from build123d import *

# Parameters (mm, degrees)
F0_W     = 30
F0_H     = 30
F1_DEPTH = 1.6
F3_DEPTH = 15
F4_DEPTH = 25


with BuildPart() as f1:
    # F0 (on Top) → F1 (new body)
    with BuildSketch(Plane.XY):
        with Locations((15, -15)):
            Rectangle(F0_W, F0_H)
    extrude(amount=F1_DEPTH)

    # F2 (on face) → F3 (join)
    with BuildSketch(Plane.XY.offset(1.6)):
        with BuildLine():
            Line((5.8029437252, -5.8029437252), (4.6715728753, -4.6715728753))
            ThreePointArc((4.6715728753, -4.6715728753), (3.5, -7.5), (4.6715728753, -10.3284271247))
            Line((4.6715728753, -10.3284271247), (5.8029437252, -9.1970562748))
            ThreePointArc((5.8029437252, -9.1970562748), (5.1, -7.5), (5.8029437252, -5.8029437252))
        make_face()
        with BuildLine():
            ThreePointArc((10.3284271247, -4.6715728753), (7.5, -3.5), (4.6715728753, -4.6715728753))
            Line((4.6715728753, -4.6715728753), (5.8029437252, -5.8029437252))
            ThreePointArc((5.8029437252, -5.8029437252), (7.5, -5.1), (9.1970562748, -5.8029437252))
            Line((9.1970562748, -5.8029437252), (10.3284271247, -4.6715728753))
        make_face()
        with BuildLine():
            ThreePointArc((11.5, -7.5), (11.19551813, -5.9692662705), (10.3284271247, -4.6715728753))
            Line((10.3284271247, -4.6715728753), (9.1970562748, -5.8029437252))
            ThreePointArc((9.1970562748, -5.8029437252), (9.717310878, -6.5815597623), (9.9, -7.5))
            ThreePointArc((9.9, -7.5), (9.717310878, -8.4184402377), (9.1970562748, -9.1970562748))
            Line((9.1970562748, -9.1970562748), (10.3284271247, -10.3284271247))
            ThreePointArc((10.3284271247, -10.3284271247), (11.19551813, -9.0307337295), (11.5, -7.5))
        make_face()
        with BuildLine():
            Line((5.8029437252, -9.1970562748), (4.6715728753, -10.3284271247))
            ThreePointArc((4.6715728753, -10.3284271247), (7.5, -11.5), (10.3284271247, -10.3284271247))
            Line((10.3284271247, -10.3284271247), (9.1970562748, -9.1970562748))
            ThreePointArc((9.1970562748, -9.1970562748), (7.5, -9.9), (5.8029437252, -9.1970562748))
        make_face()
        with BuildLine():
            ThreePointArc((18.9644660941, -18.9644660941), (17.5, -22.5), (18.9644660941, -26.0355339059))
            Line((18.9644660941, -26.0355339059), (20.095836944, -24.904163056))
            ThreePointArc((20.095836944, -24.904163056), (19.1, -22.5), (20.095836944, -20.095836944))
            Line((20.095836944, -20.095836944), (18.9644660941, -18.9644660941))
        make_face()
        with BuildLine():
            Line((24.904163056, -20.095836944), (26.0355339059, -18.9644660941))
            ThreePointArc((26.0355339059, -18.9644660941), (22.5, -17.5), (18.9644660941, -18.9644660941))
            Line((18.9644660941, -18.9644660941), (20.095836944, -20.095836944))
            ThreePointArc((20.095836944, -20.095836944), (22.5, -19.1), (24.904163056, -20.095836944))
        make_face()
        with BuildLine():
            ThreePointArc((27.5, -22.5), (27.1193976626, -20.5865828382), (26.0355339059, -18.9644660941))
            Line((26.0355339059, -18.9644660941), (24.904163056, -20.095836944))
            ThreePointArc((24.904163056, -20.095836944), (25.6411904105, -21.19887633), (25.9, -22.5))
            ThreePointArc((25.9, -22.5), (25.6411904105, -23.80112367), (24.904163056, -24.904163056))
            Line((24.904163056, -24.904163056), (26.0355339059, -26.0355339059))
            ThreePointArc((26.0355339059, -26.0355339059), (27.1193976626, -24.4134171618), (27.5, -22.5))
        make_face()
        with BuildLine():
            Line((20.095836944, -24.904163056), (18.9644660941, -26.0355339059))
            ThreePointArc((18.9644660941, -26.0355339059), (22.5, -27.5), (26.0355339059, -26.0355339059))
            Line((26.0355339059, -26.0355339059), (24.904163056, -24.904163056))
            ThreePointArc((24.904163056, -24.904163056), (22.5, -25.9), (20.095836944, -24.904163056))
        make_face()
    extrude(amount=F3_DEPTH)

    # F2 (on face) → F4 (cut)
    with BuildSketch(Plane.XY.offset(1.6)):
        with BuildLine():
            Line((26.0355339059, -11.0355339059), (22.5, -7.5))
            Line((22.5, -7.5), (18.9644660941, -11.0355339059))
            ThreePointArc((18.9644660941, -11.0355339059), (22.5, -12.5), (26.0355339059, -11.0355339059))
        make_face()
        with BuildLine():
            Line((22.5, -7.5), (18.9644660941, -3.9644660941))
            ThreePointArc((18.9644660941, -3.9644660941), (17.5, -7.5), (18.9644660941, -11.0355339059))
            Line((18.9644660941, -11.0355339059), (22.5, -7.5))
        make_face()
        with BuildLine():
            ThreePointArc((26.0355339059, -3.9644660941), (22.5, -2.5), (18.9644660941, -3.9644660941))
            Line((18.9644660941, -3.9644660941), (22.5, -7.5))
            Line((22.5, -7.5), (26.0355339059, -3.9644660941))
        make_face()
        with BuildLine():
            Line((26.0355339059, -3.9644660941), (22.5, -7.5))
            Line((22.5, -7.5), (26.0355339059, -11.0355339059))
            ThreePointArc((26.0355339059, -11.0355339059), (27.1193976626, -9.4134171618), (27.5, -7.5))
            ThreePointArc((27.5, -7.5), (27.1193976626, -5.5865828382), (26.0355339059, -3.9644660941))
        make_face()
        with BuildLine():
            Line((9.1970562748, -5.8029437252), (7.5, -7.5))
            Line((7.5, -7.5), (9.1970562748, -9.1970562748))
            ThreePointArc((9.1970562748, -9.1970562748), (9.717310878, -8.4184402377), (9.9, -7.5))
            ThreePointArc((9.9, -7.5), (9.717310878, -6.5815597623), (9.1970562748, -5.8029437252))
        make_face()
        with BuildLine():
            ThreePointArc((9.1970562748, -5.8029437252), (7.5, -5.1), (5.8029437252, -5.8029437252))
            Line((5.8029437252, -5.8029437252), (7.5, -7.5))
            Line((7.5, -7.5), (9.1970562748, -5.8029437252))
        make_face()
        with BuildLine():
            Line((7.5, -7.5), (5.8029437252, -5.8029437252))
            ThreePointArc((5.8029437252, -5.8029437252), (5.1, -7.5), (5.8029437252, -9.1970562748))
            Line((5.8029437252, -9.1970562748), (7.5, -7.5))
        make_face()
        with BuildLine():
            Line((9.1970562748, -9.1970562748), (7.5, -7.5))
            Line((7.5, -7.5), (5.8029437252, -9.1970562748))
            ThreePointArc((5.8029437252, -9.1970562748), (7.5, -9.9), (9.1970562748, -9.1970562748))
        make_face()
        with BuildLine():
            ThreePointArc((10.3284271247, -19.6715728753), (7.5, -18.5), (4.6715728753, -19.6715728753))
            Line((4.6715728753, -19.6715728753), (7.5, -22.5))
            Line((7.5, -22.5), (10.3284271247, -19.6715728753))
        make_face()
        with BuildLine():
            Line((10.3284271247, -19.6715728753), (7.5, -22.5))
            Line((7.5, -22.5), (10.3284271247, -25.3284271247))
            ThreePointArc((10.3284271247, -25.3284271247), (11.19551813, -24.0307337295), (11.5, -22.5))
            ThreePointArc((11.5, -22.5), (11.19551813, -20.9692662705), (10.3284271247, -19.6715728753))
        make_face()
        with BuildLine():
            Line((10.3284271247, -25.3284271247), (7.5, -22.5))
            Line((7.5, -22.5), (4.6715728753, -25.3284271247))
            ThreePointArc((4.6715728753, -25.3284271247), (7.5, -26.5), (10.3284271247, -25.3284271247))
        make_face()
        with BuildLine():
            Line((7.5, -22.5), (4.6715728753, -19.6715728753))
            ThreePointArc((4.6715728753, -19.6715728753), (3.5, -22.5), (4.6715728753, -25.3284271247))
            Line((4.6715728753, -25.3284271247), (7.5, -22.5))
        make_face()
        with BuildLine():
            ThreePointArc((20.095836944, -20.095836944), (19.1, -22.5), (20.095836944, -24.904163056))
            Line((20.095836944, -24.904163056), (22.5, -22.5))
            Line((22.5, -22.5), (20.095836944, -20.095836944))
        make_face()
        with BuildLine():
            Line((22.5, -22.5), (24.904163056, -20.095836944))
            ThreePointArc((24.904163056, -20.095836944), (22.5, -19.1), (20.095836944, -20.095836944))
            Line((20.095836944, -20.095836944), (22.5, -22.5))
        make_face()
        with BuildLine():
            ThreePointArc((25.9, -22.5), (25.6411904105, -21.19887633), (24.904163056, -20.095836944))
            Line((24.904163056, -20.095836944), (22.5, -22.5))
            Line((22.5, -22.5), (24.904163056, -24.904163056))
            ThreePointArc((24.904163056, -24.904163056), (25.6411904105, -23.80112367), (25.9, -22.5))
        make_face()
        with BuildLine():
            Line((22.5, -22.5), (20.095836944, -24.904163056))
            ThreePointArc((20.095836944, -24.904163056), (22.5, -25.9), (24.904163056, -24.904163056))
            Line((24.904163056, -24.904163056), (22.5, -22.5))
        make_face()
    extrude(amount=-F4_DEPTH, mode=Mode.SUBTRACT)


solid = f1.part
Geometry: final body of the model. Coordinates: model frame, mm. A direction names the side the tool comes from. Coordinates: 2 decimals unless noted, no trailing zeros. Order: outer loops, then holes, each group sorted by start corner. A loop starts at its lowest first (then second) coordinate and runs counter-clockwise, first axis right, second up.
1) Section D-D (x = 15). Return loops of the section in (y, z), then the cut area to 3 significant figures.
Result sheet:
outline: (-30, 0) - (0, 0) - (0, 1.6) - (-30, 1.6) - close
area: 48.0 mm2
2) Section B-B (x = 6.25). Return loops of the section in (y, z), then the cut area to 3 significant figures.
Result sheet:
outline: (-30, 0) - (-26.3, 0) - (-26.3, 1.6) - (-30, 1.6) - close; (-18.7, 0) - (-9.55, 0) - (-9.55, 16.6) - (-11.3, 16.6) - (-11.3, 1.6) - (-18.7, 1.6) - close; (-5.45, 0) - (0, 0) - (0, 1.6) - (-3.7, 1.6) - (-3.7, 16.6) - (-5.45, 16.6) - close
area: 81.8 mm2
3) Section C-C (y = -8.5). Return loops of the section in (x, z).
Result sheet:
outline: (0, 0) - (5.32, 0) - (5.32, 16.6) - (3.63, 16.6) - (3.63, 1.6) - (0, 1.6) - close; (9.68, 0) - (17.6, 0) - (17.6, 1.6) - (11.37, 1.6) - (11.37, 16.6) - (9.68, 16.6) - close; (27.4, 0) - (30, 0) - (30, 1.6) - (27.4, 1.6) - close
4) First-contact query: P1, Ø5, axis at y = -10.5, z = 14, coming from the -X side; P2, Ø12, axis at x = 8, y = -21, coming from the +Z side; P3, Ø1, axis at x = 19.5, y = -15, coming from the -Z side; P4, Ø1.5, axis at y = -19, z = 13, coming from the +X side. Flat tips, straight axial feed; report the tip coordinate or a pass-through.
Result sheet:
P1: stops at x = 3.53
P2: stops at z = 1.6
P3: stops at z = 0
P4: stops at x = 26.68
5) Section A-A (z = 7). Return loops of the section in (x, y).
Result sheet:
outline: circle Ø8 at (7.5, -7.5); circle Ø10 at (22.5, -22.5); hole circle Ø4.8 at (7.5, -7.5); hole circle Ø6.8 at (22.5, -22.5)
6) Set-up query: faces 1 (the flat face through (15, -15, 1.6)), 2 (the flat face through (10.1, -7.4, 16.6)). Return all of +Z, -Z, +X, -X, +Y, -Y with unobstructed straight access to the full face (end or side cutting, diameter ignored); none if empty.
Result sheet:
face 1: +Z
face 2: +Z, +X, -X, +Y, -Y
7) Ray query, probe 1 along Y at (x, z) = (6.5, 1.5); probe 2 along X at (y, z) = (-24, 1); probe 3 along Z at (x, y) = (3.5, -6). Return the intervals inside material, ascending.
Result sheet:
probe 1: y = -30 to -26.37, -18.63 to -9.68, -5.32 to 0
probe 2: x = 0 to 3.79, 11.21 to 19.45, 25.55 to 30
probe 3: z = 0 to 1.6
